Read the model definition and answer for the solid it produces. Units are mm, in the model's axes. A direction names the side the tool comes from. Round coordinates to 2 decimals unless told otherwise and drop trailing zeros. Write each loop counter-clockwise with the first axis right and the second up, starting at its lowest first coordinate (ties: lowest second). Pieces come first, ordered by that corner, then holes. Notation, with made-up numbers: (84, 45) -> (88, 45) arc R25 cw to (88, 64) -> close; hole circle Ø2 at (41, -7). An arc over 180 degrees is marked (long way). Return JSON: item names as keys, results as strings. Group by question number.
(1) A cutting plane is placed at A-A on x = 0. Give the vertices of the cut face in (y, z), then the cut area to 3 significant figures.
(2) For faces 1 (the cylindrical face through (4.191, 49.3, -100.913)), 2 (the flat face through (-17, 82, -98)), determine the directions among +Z, -Z, +X, -X, +Y, -Y from which every point of the face is accessible in a straight line to the end or side of a thin tool.
(3) A cutting plane is placed at C-C on x = -5.5. Give the vertices of the cut face in (y, z), then the cut area to 3 significant figures.
(4) Straight lines are drawn through the part: line 1 (Y direction, x = 0, z = -100.5); line 2 (Y direction, x = -15.5, z = -98.55); line 3 (Z direction, x = -15, y = 60). For each, find the intervals that lie inside material, in ascending order.
(5) Given pin 1 (8 mm diameter, centred on x = 14, y = 10.5, fed in from +Z); pin 2 (1.6 mm diameter, centred on y = 84.5, z = -99, fed in from -X); pin 3 (1.5 mm diameter, centred on x = -12.5, y = 31.5, fed in from -Z); pin 4 (3.5 mm diameter, centred on x = 0, y = 50, fed in from -Z), each flat-ended and moving along its own axis, determine where each tip first touches the part or whether it passes through.
(6) A cutting plane is placed at B-B on y = 78. Give the vertices of the cut face in (x, z).
(7) The mould has two halves that part along X. Classify faces 3 (the flat face through (-18, 18, -98)), 4 (the cylindrical face through (0.766, 51.847, -99.976)), 5 (the flat face through (-19.8, 49.6, -98)): released by +X, released by -X, zero draft, split by the parting line, or undercut.
Autodesk Inventor part; units mm, degrees
ref_plane "Work Plane1" through (0, 0, -101) normal (0, 0, -1) x (-1, 0, 0)
ref_plane "YZ Plane" through (0, 0, 0) normal (1, 0, 0) x (0, 1, 0)
ref_plane "XZ Plane" through (0, 0, 0) normal (0, 1, 0) x (-1, 0, 0)
sketch "Sketch1" plane through (0, 0, 0) normal (0, 1, 0) x (-1, 0, 0)
  arc A0 (-19.604, -97.0396) -> (19.604, -97.0396) centre (0, 0) ccw
  line L0 (19.604, -97.0396) -> (20, -99)
  line L1 (-19.604, -97.0396) -> (-20, -99)
  arc A1 (-20, -99) -> (20, -99) centre (0, 0) ccw
  line L2 (0, 0) -> (0, 18.8083) construction
  point P0 (0, -99)
  point P1 (0, -101)
  dimension "d0" = 2
  dimension "d1" = 101
  dimension "d2" = 40
  dimension "d3" = 99
extrude "Extrusion1" add sketch "Sketch1" along normal blind 100
ref_plane "Work Plane1" through (0, 0, -101) normal (0, 0, -1) x (-1, 0, 0)
sketch "Sketch2" plane through (0, 0, -101) normal (0, 0, -1) x (-1, 0, 0)
  line L0 (-20, 0) -> (20, 0)
  line L1 (20, 0) -> (20, 100)
  line L2 (-20, 100) -> (20, 100)
  line L3 (-20, 0) -> (-20, 100)
  point P0 (0, 0)
  point P1 (0, 22)
  point P2 (0, 22)
  point P3 (0, 50)
  point P4 (0, 78)
  point P5 (0, 100)
  dimension "d7" = 22
  dimension "d8" = 22
  dimension "d9" = 28
  dimension "d10" = 28
hole "Hole1" at (0, 22, -101) at (0, 50, -101) at (0, 78, -101) direction (0, 0, 1) diameter 4 end through all
sketch "Sketch3" plane through (0, 0, -101) normal (0, 0, -1) x (-1, 0, 0)
  line L0 (20, 0) -> (20, 100)
  line L1 (20, 100) -> (-20, 100)
  line L2 (20, 0) -> (-20, 0)
  line L3 (20, 89) -> (15, 89)
  line L4 (15, 89) -> (15, 82)
  line L5 (15, 82) -> (20, 82)
  line L6 (20, 18) -> (15, 18)
  line L7 (15, 18) -> (15, 11)
  line L8 (15, 11) -> (20, 11)
  point P0 (0, 0)
  point P1 (0, 52)
  point P2 (0, 48)
  dimension "d18" = 7
  dimension "d19" = 5
  dimension "d20" = 11
  dimension "d21" = 5
  dimension "d22" = 11
  dimension "d23" = 7
extrude "Extrusion2" cut sketch "Sketch3" against normal up to surface
properties part number "214,2"
Checks:
{
 "1": {"outline": "(0, -101) -> (20, -101) -> (20, -99) -> (0, -99) -> close; (24, -101) -> (48, -101) -> (48, -99) -> (24, -99) -> close; (52, -101) -> (76, -101) -> (76, -99) -> (52, -99) -> close; (80, -101) -> (100, -101) -> (100, -99) -> (80, -99) -> close", "area": "176 mm^2"},
 "2": {"face 1": "-Z, +Y, -Y", "face 2": "+Z, -Z, -X"},
 "3": {"outline": "(0, -100.85) -> (100, -100.85) -> (100, -98.85) -> (0, -98.85) -> close", "area": "200 mm^2"},
 "4": {"line 1": "y = 0 to 20, 24 to 48, 52 to 76, 80 to 100", "line 2": "y = 0 to 11, 18 to 82, 89 to 100", "line 3": "z = -99.88 to -97.86"},
 "5": {"pin 1": "stops at z = -97.35", "pin 2": "stops at x = -15", "pin 3": "stops at z = -100.31", "pin 4": "passes through"},
 "6": {"outline": "(-20, -99) arc R101 ccw to (-2, -100.98) -> (-2, -98.98) arc R99 cw to (-19.6, -97.04) -> close; (2, -100.98) arc R101 ccw to (20, -99) -> (19.6, -97.04) arc R99 cw to (2, -98.98) -> close"},
 "7": {"face 3": "zero draft", "face 4": "undercut", "face 5": "released by -X"}
}
